```python
from build123d import *

# Parameters (mm, degrees)
BOSS_EXTRUDE1_DEPTH = 10
SKETCH2_W           = 10
SKETCH2_H           = 10
BOSS_EXTRUDE2_DEPTH = 10


with BuildPart() as part:
    # Sketch1 → Boss-Extrude1 (new body)
    with BuildSketch(Plane(origin=(0, 0, 0), x_dir=(0, 0, -1), z_dir=(1, 0, 0))):
        with BuildLine():
            Line((-8.804034582, 5), (12.995965418, 5))
            ThreePointArc((12.995965418, 5), (23.602567136, 9.393398282), (27.995965418, 20))
            Line((27.995965418, 20), (27.995965418, -20))
            ThreePointArc((27.995965418, -20), (23.602567136, -9.393398282), (12.995965418, -5))
            Line((12.995965418, -5), (-8.804034582, -5))
            ThreePointArc((-8.804034582, -5), (-19.4106363, -9.393398282), (-23.804034582, -20))
            Line((-23.804034582, -20), (-23.804034582, 20))
            ThreePointArc((-23.804034582, 20), (-19.4106363, 9.393398282), (-8.804034582, 5))
        make_face()
    extrude(amount=BOSS_EXTRUDE1_DEPTH)

    # Sketch2 → Boss-Extrude2 (add)
    with BuildSketch(Plane.XY.offset(23.804034582)):
        with Locations((5, 0)):
            Rectangle(SKETCH2_W, SKETCH2_H)
    boss_extrude2 = extrude(amount=BOSS_EXTRUDE2_DEPTH)

    # Mirror1: Boss-Extrude2 across plane
    add(boss_extrude2.mirror(Plane(origin=(0, 0, -2.095965418), x_dir=(1, 0, 0), z_dir=(0, 0, -1))))


solid = part.part
```
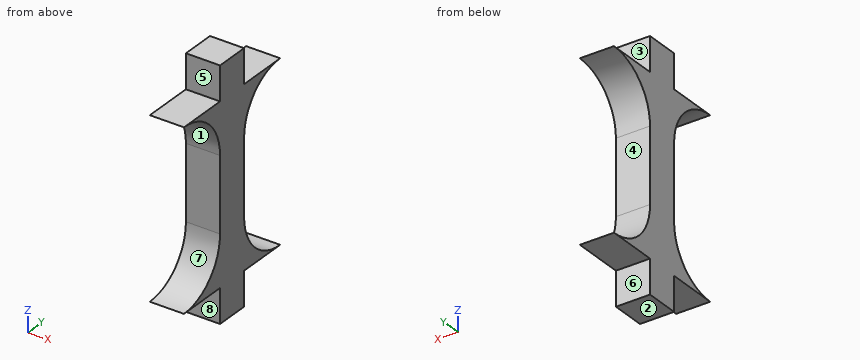
Geometry: final body of the model. Coordinates: model frame, mm. Face numbers are marked on the shaded views. A direction names the side the tool comes from. Round coordinates to 2 decimals unless told otherwise and drop trailing zeros. Loops run counter-clockwise (first coordinate to the right, second up) from the corner with the lowest first, then second, coordinate; pieces in that order, holes last. Notation, with made-up numbers: (-32.5, -15.75) -> (2.5, -15.75) arc R24 ccw to (2.5, -2.75) -> close; hole circle Ø9 at (-20.75, 3). An arc over 180 degrees is marked (long way). Use one line per item in the form item = value. Start each with the question number.
1) Section B-B on x = 5.25. Output: boundary loops of the cut face in (y, z).
2) Draft query along Z for the marked faces 1, 2 and 3. Return one class per face: released by +Z, released by -Z, zero draft, split by the parting line, or undercut.
3) First-contact query: P1, Ø2, axis at x = 4, z = 15.5, coming from the -Y side; P2, Ø3, axis at x = 3.5, z = 29, coming from the -Y side; P3, Ø5, axis at x = 6, z = -7, coming from the +Y side; P4, Ø3, axis at y = -12, z = 26.5, coming from the +X side. Flat tips, straight axial feed; report the tip coordinate or a pass-through.
4) Section A-A on y = -10. Output: boundary loops of the cut face in (x, z).
5) Line query: L1, parallel to Y at x = 2.5, z = -7.5; L2, parallel to Z at x = 7.5, y = 15.5; L3, parallel to Z at x = 1.5, y = -8.5. Output: solid intervals per line, ascending.
6) Section D-D on z = 7. Output: boundary loops of the cut face in (x, y).
7) Access query for the marked faces 4, 5, 6, 7 and 8. Directions: +Z, -Z, +X, -X, +Y, -Y. A direction counts if a zero-diameter tool reaches every point of the face in a straight line with its end or side. Return the directions, or none.
8) Section C-C on y = 14.5. Output: boundary loops of the cut face in (x, z), then the cut area to 3 significant figures.
Response:
q1.outline = (-20, -28) -> (-5, -28) -> (-5, -38) -> (5, -38) -> (5, -28) -> (20, -28) arc R15 cw to (5, -13) -> (5, 8.8) arc R15 cw to (20, 23.8) -> (5, 23.8) -> (5, 33.8) -> (-5, 33.8) -> (-5, 23.8) -> (-20, 23.8) arc R15 cw to (-5, 8.8) -> (-5, -13) arc R15 cw to start
q2.face_1 = undercut
q2.face_2 = released by -Z
q2.face_3 = zero draft
q3.P1 = -7.12
q3.P2 = -5
q3.P3 = 5
q3.P4 = through
q4.outline = (0, -28) -> (10, -28) -> (10, -24.18) -> (0, -24.18) -> close; (0, 19.98) -> (10, 19.98) -> (10, 23.8) -> (0, 23.8) -> close
q5.L1 = -5 to 5
q5.L2 = -28 to -27.31, 23.11 to 23.8
q5.L3 = -28 to -22.63, 18.43 to 23.8
q6.outline = (0, -5) -> (10, -5) -> (10, 5) -> (0, 5) -> close
q7.face_4 = +X, -X, +Y
q7.face_5 = +Z, +X, -X, -Y
q7.face_6 = -Z, +X, -X, +Y
q7.face_7 = +X, -X, -Y
q7.face_8 = -Z, +X, -X, -Y
q8.outline = (0, -28) -> (10, -28) -> (10, -26.95) -> (0, -26.95) -> close; (0, 22.76) -> (10, 22.76) -> (10, 23.8) -> (0, 23.8) -> close
q8.area = 20.9 mm^2
